Here's how the part is built. I have some questions about the finished solid (model axes, mm). A direction names the side the tool comes from. Round coordinates to 2 decimals unless told otherwise and drop trailing zeros. Write each loop counter-clockwise with the first axis right and the second up, starting at its lowest first coordinate (ties: lowest second). Pieces come first, ordered by that corner, then holes. Notation, with made-up numbers: M 57,-10.75 L 77,-10.75 A29 ccw 77,27.25 Z; hole C -9,-3.5 d8. An arc over 180 degrees is marked long. Use one line per item in the form item = value. Start each with the question number.
Q1. For faces 5 (the face through (-3.4, -2.2, -192.5)), 6 (the face through (0, -5.835, 3)), 7 (the face through (5.835, 0, 3)), 8 (the face through (-5.835, 0, 3)), which set-ups out of +Z, -Z, +X, -X, +Y, -Y let a thin tool reach every point of the face, with its end or its side?
Q2. I'm going to push flat-ended pins straight in: pin 1 Ø1.5 at (x, z) = (-3, 103.5) entering from -Y; pin 2 Ø0.6 at (y, z) = (-14, -48.5) entering from -X; pin 3 Ø6 at (x, y) = (-11.5, -4) entering from +Z; pin 4 Ø1.5 at (y, z) = (-1, 78.5) entering from +X. Where does each tip first touch, or does it pass through?
Q3. I need wall thicknesses on line 1 along Y through (x, z) = (12.5, 31.5); line 2 along X through (y, z) = (13.5, 48); line 3 along Y through (x, z) = (0, 22.5). Which ranges of each line are inside material? Lowest first, please. Write a range as from..to.
Q4. We'd pull the mould along Y, two halves only. Please class faces 1 (the face through (-9, -15, 3)), 2 (the face through (15, 9, 3)), 3 (the face through (3.367, 1.06, -2.695)), 4 (the face through (0, 5.835, 3)): +Y half, -Y half, draft (parallel to the pull), parting line (faces both ways), or undercut.
Q5. I want a section at C-C on z = -59.5. State how many separate pieces and enclosed holes the cut face has, and give its area (3 significant figures).
Q6. I want a section at A-A on y = 0. List the corners of the cut face in (x, z) for me, and give its area (3 significant figures).
```python
from build123d import *

# Parameters (mm, degrees)
SKETCH1_R           = 3.52998588
BOSS_EXTRUDE1_DEPTH = 192.5


with BuildPart() as part:
    # Sketch1 → Boss-Extrude1 (new body, symmetric)
    with BuildSketch(Plane.XY):
        with BuildLine():
            Line((14.49994, -4), (13.24247465, -4))
            ThreePointArc((13.24247465, -4), (12.88892126, -4.146446609), (12.74247465, -4.5))
            Line((12.74247465, -4.5), (12.74247465, -7.732519321))
            ThreePointArc((12.74247465, -7.732519321), (12.602449697, -8.097296796), (12.242781236, -8.249967))
            Line((12.242781236, -8.249967), (10.260188032, -8.249967))
            ThreePointArc((10.260188032, -8.249967), (10.068847082, -8.211906919), (9.906636056, -8.103520976))
            Line((9.906636056, -8.103520976), (5.981117769, -4.178002689))
            ThreePointArc((5.981117769, -4.178002689), (5.872731827, -4.015791664), (5.834671745, -3.824450713))
            Line((5.834671745, -3.824450713), (5.834671745, -1.01249595))
            Line((5.834671745, -1.01249595), (5.834671745, 0.88749645))
            Line((5.834671745, 0.88749645), (5.834671745, 3.824450713))
            ThreePointArc((5.834671745, 3.824450713), (5.872731827, 4.015791664), (5.981117769, 4.178002689))
            Line((5.981117769, 4.178002689), (9.906636056, 8.103520976))
            ThreePointArc((9.906636056, 8.103520976), (10.068847082, 8.211906919), (10.260188032, 8.249967))
            Line((10.260188032, 8.249967), (12.242781236, 8.249967))
            ThreePointArc((12.242781236, 8.249967), (12.602449697, 8.097296796), (12.74247465, 7.732519321))
            Line((12.74247465, 7.732519321), (12.74247465, 4.5))
            ThreePointArc((12.74247465, 4.5), (12.88892126, 4.146446609), (13.24247465, 4))
            Line((13.24247465, 4), (14.49994, 4))
            ThreePointArc((14.49994, 4), (14.853493391, 4.146446609), (14.99994, 4.5))
            Line((14.99994, 4.5), (14.99994, 12.999948))
            ThreePointArc((14.99994, 12.999948), (14.414155906, 14.414155906), (12.999948, 14.99994))
            Line((12.999948, 14.99994), (4.5, 14.99994))
            ThreePointArc((4.5, 14.99994), (4.146446609, 14.853493391), (4, 14.49994))
            Line((4, 14.49994), (4, 13.24247465))
            ThreePointArc((4, 13.24247465), (4.146446609, 12.88892126), (4.5, 12.74247465))
            Line((4.5, 12.74247465), (7.732519321, 12.74247465))
            ThreePointArc((7.732519321, 12.74247465), (8.097296796, 12.602449697), (8.249967, 12.242781236))
            Line((8.249967, 12.242781236), (8.249967, 10.260188032))
            ThreePointArc((8.249967, 10.260188032), (8.211906919, 10.068847082), (8.103520976, 9.906636056))
            Line((8.103520976, 9.906636056), (4.178002689, 5.981117769))
            ThreePointArc((4.178002689, 5.981117769), (4.015791664, 5.872731827), (3.824450713, 5.834671745))
            Line((3.824450713, 5.834671745), (0.9499962, 5.834671745))
            Line((0.9499962, 5.834671745), (-0.9499962, 5.834671745))
            Line((-0.9499962, 5.834671745), (-3.824450713, 5.834671745))
            ThreePointArc((-3.824450713, 5.834671745), (-4.015791664, 5.872731827), (-4.178002689, 5.981117769))
            Line((-4.178002689, 5.981117769), (-8.103520976, 9.906636056))
            ThreePointArc((-8.103520976, 9.906636056), (-8.211906919, 10.068847082), (-8.249967, 10.260188032))
            Line((-8.249967, 10.260188032), (-8.249967, 12.242781236))
            ThreePointArc((-8.249967, 12.242781236), (-8.097296796, 12.602449697), (-7.732519321, 12.74247465))
            Line((-7.732519321, 12.74247465), (-4.5, 12.74247465))
            ThreePointArc((-4.5, 12.74247465), (-4.146446609, 12.88892126), (-4, 13.24247465))
            Line((-4, 13.24247465), (-4, 14.49994))
            ThreePointArc((-4, 14.49994), (-4.146446609, 14.853493391), (-4.5, 14.99994))
            Line((-4.5, 14.99994), (-12.999948, 14.99994))
            ThreePointArc((-12.999948, 14.99994), (-14.414155906, 14.414155906), (-14.99994, 12.999948))
            Line((-14.99994, 12.999948), (-14.99994, 4.5))
            ThreePointArc((-14.99994, 4.5), (-14.853493391, 4.146446609), (-14.49994, 4))
            Line((-14.49994, 4), (-13.24247465, 4))
            ThreePointArc((-13.24247465, 4), (-12.88892126, 4.146446609), (-12.74247465, 4.5))
            Line((-12.74247465, 4.5), (-12.74247465, 7.732519321))
            ThreePointArc((-12.74247465, 7.732519321), (-12.602449697, 8.097296796), (-12.242781236, 8.249967))
            Line((-12.242781236, 8.249967), (-10.260188032, 8.249967))
            ThreePointArc((-10.260188032, 8.249967), (-10.068847082, 8.211906919), (-9.906636056, 8.103520976))
            Line((-9.906636056, 8.103520976), (-5.981117769, 4.178002689))
            ThreePointArc((-5.981117769, 4.178002689), (-5.872731827, 4.015791664), (-5.834671745, 3.824450713))
            Line((-5.834671745, 3.824450713), (-5.834671745, 0.88749645))
            Line((-5.834671745, 0.88749645), (-5.834671745, -1.01249595))
            Line((-5.834671745, -1.01249595), (-5.834671745, -3.824450713))
            ThreePointArc((-5.834671745, -3.824450713), (-5.872731827, -4.015791664), (-5.981117769, -4.178002689))
            Line((-5.981117769, -4.178002689), (-9.906636056, -8.103520976))
            ThreePointArc((-9.906636056, -8.103520976), (-10.068847082, -8.211906919), (-10.260188032, -8.249967))
            Line((-10.260188032, -8.249967), (-12.242781236, -8.249967))
            ThreePointArc((-12.242781236, -8.249967), (-12.602449697, -8.097296796), (-12.74247465, -7.732519321))
            Line((-12.74247465, -7.732519321), (-12.74247465, -4.5))
            ThreePointArc((-12.74247465, -4.5), (-12.88892126, -4.146446609), (-13.24247465, -4))
            Line((-13.24247465, -4), (-14.49994, -4))
            ThreePointArc((-14.49994, -4), (-14.853493391, -4.146446609), (-14.99994, -4.5))
            Line((-14.99994, -4.5), (-14.99994, -12.999948))
            ThreePointArc((-14.99994, -12.999948), (-14.414155906, -14.414155906), (-12.999948, -14.99994))
            Line((-12.999948, -14.99994), (-4.5, -14.99994))
            ThreePointArc((-4.5, -14.99994), (-4.146446609, -14.853493391), (-4, -14.49994))
            Line((-4, -14.49994), (-4, -13.24247465))
            ThreePointArc((-4, -13.24247465), (-4.146446609, -12.88892126), (-4.5, -12.74247465))
            Line((-4.5, -12.74247465), (-7.732519321, -12.74247465))
            ThreePointArc((-7.732519321, -12.74247465), (-8.097296796, -12.602449697), (-8.249967, -12.242781236))
            Line((-8.249967, -12.242781236), (-8.249967, -10.260188032))
            ThreePointArc((-8.249967, -10.260188032), (-8.211906919, -10.068847082), (-8.103520976, -9.906636056))
            Line((-8.103520976, -9.906636056), (-4.178002689, -5.981117769))
            ThreePointArc((-4.178002689, -5.981117769), (-4.015791664, -5.872731827), (-3.824450713, -5.834671745))
            Line((-3.824450713, -5.834671745), (-0.9499962, -5.834671745))
            Line((-0.9499962, -5.834671745), (0.9499962, -5.834671745))
            Line((0.9499962, -5.834671745), (3.824450713, -5.834671745))
            ThreePointArc((3.824450713, -5.834671745), (4.015791664, -5.872731827), (4.178002689, -5.981117769))
            Line((4.178002689, -5.981117769), (8.103520976, -9.906636056))
            ThreePointArc((8.103520976, -9.906636056), (8.211906919, -10.068847082), (8.249967, -10.260188032))
            Line((8.249967, -10.260188032), (8.249967, -12.242781236))
            ThreePointArc((8.249967, -12.242781236), (8.097296796, -12.602449697), (7.732519321, -12.74247465))
            Line((7.732519321, -12.74247465), (4.5, -12.74247465))
            ThreePointArc((4.5, -12.74247465), (4.146446609, -12.88892126), (4, -13.24247465))
            Line((4, -13.24247465), (4, -14.49994))
            ThreePointArc((4, -14.49994), (4.146446609, -14.853493391), (4.5, -14.99994))
            Line((4.5, -14.99994), (12.999948, -14.99994))
            ThreePointArc((12.999948, -14.99994), (14.414155906, -14.414155906), (14.99994, -12.999948))
            Line((14.99994, -12.999948), (14.99994, -4.5))
            ThreePointArc((14.99994, -4.5), (14.853493391, -4.146446609), (14.49994, -4))
        make_face()
        Circle(SKETCH1_R, mode=Mode.SUBTRACT)
        with BuildLine():
            Line((-12.6999492, -13.6999452), (-9.880960476, -13.6999452))
            ThreePointArc((-9.880960476, -13.6999452), (-9.61155387, -13.58835333), (-9.499962, -13.318946724))
            Line((-9.499962, -13.318946724), (-9.499962, -9.87996048))
            ThreePointArc((-9.499962, -9.87996048), (-9.611260978, -9.611260978), (-9.87996048, -9.499962))
            Line((-9.87996048, -9.499962), (-13.318946724, -9.499962))
            ThreePointArc((-13.318946724, -9.499962), (-13.58835333, -9.61155387), (-13.6999452, -9.880960476))
            Line((-13.6999452, -9.880960476), (-13.6999452, -12.6999492))
            ThreePointArc((-13.6999452, -12.6999492), (-13.407053153, -13.407053153), (-12.6999492, -13.6999452))
        make_face(mode=Mode.SUBTRACT)
        with BuildLine():
            Line((13.6999452, -12.6999492), (13.6999452, -9.880960476))
            ThreePointArc((13.6999452, -9.880960476), (13.58835333, -9.61155387), (13.318946724, -9.499962))
            Line((13.318946724, -9.499962), (9.87996048, -9.499962))
            ThreePointArc((9.87996048, -9.499962), (9.611260978, -9.611260978), (9.499962, -9.87996048))
            Line((9.499962, -9.87996048), (9.499962, -13.318946724))
            ThreePointArc((9.499962, -13.318946724), (9.61155387, -13.58835333), (9.880960476, -13.6999452))
            Line((9.880960476, -13.6999452), (12.6999492, -13.6999452))
            ThreePointArc((12.6999492, -13.6999452), (13.407053153, -13.407053153), (13.6999452, -12.6999492))
        make_face(mode=Mode.SUBTRACT)
        with BuildLine():
            Line((9.87996048, 9.499962), (13.318946724, 9.499962))
            ThreePointArc((13.318946724, 9.499962), (13.58835333, 9.61155387), (13.6999452, 9.880960476))
            Line((13.6999452, 9.880960476), (13.6999452, 12.6999492))
            ThreePointArc((13.6999452, 12.6999492), (13.407053153, 13.407053153), (12.6999492, 13.6999452))
            Line((12.6999492, 13.6999452), (9.880960476, 13.6999452))
            ThreePointArc((9.880960476, 13.6999452), (9.61155387, 13.58835333), (9.499962, 13.318946724))
            Line((9.499962, 13.318946724), (9.499962, 9.87996048))
            ThreePointArc((9.499962, 9.87996048), (9.611260978, 9.611260978), (9.87996048, 9.499962))
        make_face(mode=Mode.SUBTRACT)
        with BuildLine():
            Line((-13.6999452, 12.6999492), (-13.6999452, 9.880960476))
            ThreePointArc((-13.6999452, 9.880960476), (-13.58835333, 9.61155387), (-13.318946724, 9.499962))
            Line((-13.318946724, 9.499962), (-9.87996048, 9.499962))
            ThreePointArc((-9.87996048, 9.499962), (-9.611260978, 9.611260978), (-9.499962, 9.87996048))
            Line((-9.499962, 9.87996048), (-9.499962, 13.318946724))
            ThreePointArc((-9.499962, 13.318946724), (-9.61155387, 13.58835333), (-9.880960476, 13.6999452))
            Line((-9.880960476, 13.6999452), (-12.6999492, 13.6999452))
            ThreePointArc((-12.6999492, 13.6999452), (-13.407053153, 13.407053153), (-13.6999452, 12.6999492))
        make_face(mode=Mode.SUBTRACT)
    extrude(amount=BOSS_EXTRUDE1_DEPTH, both=True)


solid = part.part
```
Reported:
q1.face_5 = -Z, +X, -X, +Y, -Y
q1.face_6 = +Z, -Z, -Y
q1.face_7 = +Z, -Z, +X
q1.face_8 = +Z, -Z, -X
q2.pin_1 = -5.83
q2.pin_2 = -14.87
q2.pin_3 = 192.5
q2.pin_4 = 5.83
q3.line_1 = -15..-13.7, -9.5..-8.18, 8.18..9.5, 13.7..15
q3.line_2 = -14.94..-13.3, -9.55..-4, 4..9.55, 13.3..14.94
q3.line_3 = -5.83..-3.53, 3.53..5.83
q4.face_1 = -Y half
q4.face_2 = draft
q4.face_3 = undercut
q4.face_4 = +Y half
q5.separate_pieces = 1
q5.enclosed_holes = 5
q5.area = 331 mm^2
q6.outline = M -5.83,-192.5 L -3.53,-192.5 L -3.53,192.5 L -5.83,192.5 Z; M 3.53,-192.5 L 5.83,-192.5 L 5.83,192.5 L 3.53,192.5 Z
q6.area = 1,770 mm^2
